Here's how the part is built. I have some questions about the finished solid (model axes, mm). A direction names the side the tool comes from. Give positions to 0.01 mm unless a question says otherwise; leave off trailing zeros. Write each loop counter-clockwise with the first axis right and the second up, starting at its lowest first coordinate (ties: lowest second). Pieces come first, ordered by that corner, then holes. Notation, with made-up numbers: (61, 72.25) - (71, 72.25) arc R26 ccw to (71, 94.25) - close; hole circle Ø8 at (16.25, 41.5). An arc over 180 degrees is marked (long way). One line per item, written item: value. Start each with the question number.
1) Imagine slicing it at A-A on x = 16. Write out the boundary of the cut face in (y, z).
2) On a 3-axis mill with a long thin cutter (end or side, diameter ignored), from which of +Z, -Z, +X, -X, +Y, -Y can I reach the whole of each face in a straight line? I mean faces 3 (the flat face through (38, 1, 33.5)), 4 (the flat face through (30, 0, 17)). Say none if no direction works.
3) I'm going to push flat-ended pins straight in: P1, Ø4.5, axis at x = 5, z = 30, coming from the +Y side; P2, Ø3, axis at x = 18, z = 30, coming from the -Y side. Where does each tip first touch, or does it pass through?
4) Please list where these lines run through material, in increasing order: L1, parallel to Z at x = 22, y = 1.05; L2, parallel to X at y = 0.45, z = 9.5; L3, parallel to Z at x = 55, y = 2.05. Write a range as [from, to].
5) Imagine slicing it at C-C on x = 55. Write out the boundary of the cut face in (y, z), plus the area to 3 significant figures.
6) Imagine slicing it at B-B on y = 0.9. Count the separate pieces of the cut face and the enclosed holes in it, plus the area to 3 significant figures.
7) We'd pull the mould along X, two halves only. Please class faces 1 (the cylindrical face through (6.48, 1.48, 32.32)), 2 (the flat face through (30, 3, 17)): +X half, -X half, draft (parallel to the pull), parting line (faces both ways), or undercut.
from build123d import *

# Parameters (mm, degrees)
SKETCH_W      = 60
SKETCH_H      = 3
PAD_DEPTH     = 35
SKETCH001_R   = 1.5
SKETCH001_R_2 = 2
SKETCH001_R_3 = 2.75
SKETCH001_R_4 = 1
SKETCH001_W   = 4
SKETCH001_H   = 7
POCKET_DEPTH  = 3


with BuildPart() as part:
    # Sketch → Pad (new body)
    with BuildSketch(Plane.XY):
        with Locations((30, 1.5)):
            Rectangle(SKETCH_W, SKETCH_H)
    extrude(amount=PAD_DEPTH)

    # Sketch001 → Pocket (cut)
    with BuildSketch(Plane.XZ):
        with Locations((22, 10)):
            Circle(SKETCH001_R)
        with Locations((28, 10)):
            Circle(SKETCH001_R_2)
        with Locations((22, 16)):
            Circle(SKETCH001_R_2)
        with Locations((16, 10)):
            Circle(SKETCH001_R_2)
        with Locations((22, 4)):
            Circle(SKETCH001_R_2)
        with Locations((5, 30)):
            Circle(SKETCH001_R_3)
        with Locations((55, 30)):
            Circle(SKETCH001_R_3)
        with Locations((14, 30)):
            Circle(SKETCH001_R_4)
        with Locations((18, 30)):
            Circle(SKETCH001_R_4)
        with Locations((26, 30)):
            Circle(SKETCH001_R_4)
        with Locations((30, 30)):
            Circle(SKETCH001_R_4)
        with Locations((34, 30)):
            Circle(SKETCH001_R_4)
        with Locations((42, 30)):
            Circle(SKETCH001_R_4)
        with Locations((46, 30)):
            Circle(SKETCH001_R_4)
        with Locations((45.6, 15)):
            Circle(SKETCH001_R)
        with Locations((45.6, 4.8)):
            Circle(SKETCH001_R)
        with Locations((22, 30)):
            Rectangle(SKETCH001_W, SKETCH001_H)
        with Locations((38, 30)):
            Rectangle(SKETCH001_W, SKETCH001_H)
    extrude(amount=-POCKET_DEPTH, mode=Mode.SUBTRACT)


solid = part.part
Numbers:
1. outline: (0, 0) - (3, 0) - (3, 8) - (0, 8) - close; (0, 12) - (3, 12) - (3, 35) - (0, 35) - close
2. face 3: +Y, -Y
2. face 4: +Z, -Z, +X, -X, -Y
3. P1: through
3. P2: y = 0
4. L1: [0, 2], [6, 8.5], [11.5, 14], [18, 26.5], [33.5, 35]
4. L2: [0, 14.06], [17.94, 20.59], [23.41, 26.06], [29.94, 60]
4. L3: [0, 27.25], [32.75, 35]
5. outline: (0, 0) - (3, 0) - (3, 27.25) - (0, 27.25) - close; (0, 32.75) - (3, 32.75) - (3, 35) - (0, 35) - close
5. area: 88.5 mm^2
6. separate pieces: 1
6. enclosed holes: 18
6. area: 1,900 mm^2
7. face 1: undercut
7. face 2: draft
